For this review, take the finished solid that the model builds, in its own axes (mm). Coordinates: 2 decimals unless noted, no trailing zeros. Loops run counter-clockwise (first coordinate to the right, second up) from the corner with the lowest first, then second, coordinate; pieces in that order, holes last. Notation, with made-up numbers: (52, -30) - (87, -30) arc R16 ccw to (87, -23) - close; hole circle Ø4 at (62.5, 7.25). An arc over 180 degrees is marked (long way). Answer as a JSON object with one key per item and string values. Group by question number.
Item 1: We need section D-D (y = 5). State how many separate pieces and enclosed holes the cut face has, then the cut area to 3 significant figures.
Item 2: Clearance check with flat-ended pins moving along their axes: pin 1 (3.5 mm diameter, centred on y = 4.5, z = -31.5, fed in from -X); pin 2 (5 mm diameter, centred on y = 5, z = -90.52, fed in from -X); pin 3 (0.6 mm diameter, centred on x = -4.5, y = 3, fed in from +Z). State where each tip first meets the part, or that it passes through.
Item 3: We need section C-C (z = -28). Give the boundary of the cut face in (x, y), then the cut area to 3 significant figures.
Item 4: We need section B-B (z = -9). Give the boundary of the cut face in (x, y), then the cut area to 3 significant figures.
Item 5: To check wall thickness, follow line 1 (Y direction, x = 2.95, z = -90.52); line 2 (X direction, y = 3.5, z = -92); line 3 (X direction, y = 5.5, z = -7). State the ranges of each line that lie inside material, in increasing order.
Item 6: We need section A-A (z = -90.52). Give the boundary of the cut face in (x, y), then the cut area to 3 significant figures.
from build123d import *

# Parameters (mm, degrees)
SKETCH1_W                        = 5.5
SKETCH1_H                        = 11
MAIN_BASE_DEPTH                  = 96.52
SIDE_CUT_OUT_DEPTH               = 84.52
TOP_RUBBER_BAND_CUT_OUT_DEPTH    = 98.300361767
BOTTOM_RUBBER_BAND_CUT_OUT_DEPTH = 98.300361767
SKETCH6_W                        = 1.75
SKETCH6_H                        = 11
MOTOR_PULLEY_CUT_OUT_DEPTH       = 12
SKETCH7_W                        = 1.75
SKETCH7_H                        = 11
PULLEY_CUT_OUT_DEPTH             = 10
SKETCH11_R                       = 1.5
MOTOR_SHAFT_CUT_OUT_DEPTH        = 98.217143036
SKETCH17_W                       = 3.14
SKETCH17_H                       = 2.8
MOUNTING_POINTS_DEPTH            = 8.5
MOUNTING_POINTS_DRAFT            = -1.348
MOUNTING_POINTS_PROFILE_2_DEPTH  = 8.5
MOUNTING_POINTS_PROFILE_2_DRAFT  = -1.348
SKETCH13_W                       = 1
SKETCH13_H                       = 0.5
BOSS_EXTRUDE3_DEPTH              = 12
RAIL_CHAMFER_SIZE                = 0.5


with BuildPart() as part:
    # Sketch1 → main_base (new body)
    with BuildSketch(Plane.XY):
        with Locations((2.75, 5.5)):
            Rectangle(SKETCH1_W, SKETCH1_H)
    extrude(amount=-MAIN_BASE_DEPTH)

    # Sketch3 → side_cut_out (cut)
    with BuildSketch(Plane.XY):
        Polygon((5.5, 9), (3.5, 7), (3.5, 0), (5.5, 0), align=None)
    extrude(amount=-SIDE_CUT_OUT_DEPTH, mode=Mode.SUBTRACT)

    # Sketch4 → top_rubber_band_cut_out (cut, through all)
    with BuildSketch(Plane.XY):
        Polygon((0, 7.3), (0, 11), (2.7, 11), (2.7, 10), align=None)
    extrude(amount=-TOP_RUBBER_BAND_CUT_OUT_DEPTH, mode=Mode.SUBTRACT)

    # Sketch5 → bottom_rubber_band_cut_out (cut, through all)
    with BuildSketch(Plane.XY):
        Polygon((2, 0), (0, 2), (0, 0), align=None)
    extrude(amount=-BOTTOM_RUBBER_BAND_CUT_OUT_DEPTH, mode=Mode.SUBTRACT)

    # Sketch6 → motor_pulley_cut_out (cut)
    with BuildSketch(Plane(origin=(0, 0, -96.52), x_dir=(-1, 0, 0), z_dir=(0, 0, -1))):
        with Locations((-0.875, 5.5)):
            Rectangle(SKETCH6_W, SKETCH6_H)
    extrude(amount=-MOTOR_PULLEY_CUT_OUT_DEPTH, mode=Mode.SUBTRACT)

    # Sketch7 → pulley_cut_out (cut)
    with BuildSketch(Plane.XY):
        with Locations((0.875, 5.5)):
            Rectangle(SKETCH7_W, SKETCH7_H)
    extrude(amount=-PULLEY_CUT_OUT_DEPTH, mode=Mode.SUBTRACT)

    # Sketch10 → half_circle_cut_out (revolve, cut)
    with BuildSketch(Plane(origin=(0, 5, 0), x_dir=(1, 0, 0), z_dir=(0, 1, 0))):
        with BuildLine():
            Line((1.5, 5), (1.5, 3.75))
            ThreePointArc((1.5, 3.75), (2.383883476, 4.116116524), (2.75, 5))
            Line((2.75, 5), (1.5, 5))
        make_face()
    revolve(axis=Axis((2.75, 5, -5), (-1, 0, 0)), mode=Mode.SUBTRACT)

    # Sketch11 → motor_shaft_cut_out (cut, through all)
    with BuildSketch(Plane.ZY.offset(-1.75)):
        with Locations((-90.52, 5)):
            Circle(SKETCH11_R)
    extrude(amount=-MOTOR_SHAFT_CUT_OUT_DEPTH, mode=Mode.SUBTRACT)


with BuildPart() as mounting_points_tool:
    # Sketch17 → mounting_points (with draft: the straight prism first)
    with BuildSketch(Plane.XZ):
        with Locations((4.13, -0.15)):
            Rectangle(SKETCH17_W, SKETCH17_H)
    extrude(amount=-MOUNTING_POINTS_DEPTH)
    # mounting_points: the draft: its side faces are tilted about the plane it starts from
    mounting_points_sides = [mounting_points_tool.faces().sort_by_distance(p)[0] for p in [
        (4.13, 4.25, 1.25),
        (2.56, 4.25, -0.15),
        (4.13, 4.25, -1.55),
        (5.7, 4.25, -0.15),
    ]]
    draft(mounting_points_sides, Plane.XZ, MOUNTING_POINTS_DRAFT)


with BuildPart() as part_1:
    add(part.part)

    # mounting_points: cut by mounting_points_tool
    add(mounting_points_tool.part, mode=Mode.SUBTRACT)


with BuildPart() as mounting_points_profile_2_tool:
    # Sketch17 → mounting_points profile 2 (with draft: the straight prism first)
    with BuildSketch(Plane.XZ):
        with Locations((4.13, -96.37)):
            Rectangle(SKETCH17_W, SKETCH17_H)
    extrude(amount=-MOUNTING_POINTS_PROFILE_2_DEPTH)
    # mounting_points profile 2: the draft: its side faces are tilted about the plane it starts from
    mounting_points_profile_2_sides = [mounting_points_profile_2_tool.faces().sort_by_distance(p)[0] for p in [
        (4.13, 4.25, -97.77),
        (5.7, 4.25, -96.37),
        (4.13, 4.25, -94.97),
        (2.56, 4.25, -96.37),
    ]]
    draft(mounting_points_profile_2_sides, Plane.XZ, MOUNTING_POINTS_PROFILE_2_DRAFT)


with BuildPart() as part_2:
    add(part_1.part)

    # mounting_points profile 2: cut by mounting_points_profile_2_tool
    add(mounting_points_profile_2_tool.part, mode=Mode.SUBTRACT)

    # final_mirror: part across plane


with BuildPart() as part_3:
    add(part_2.part)
    add(part_2.part.mirror(Plane(origin=(0, 0, 0), x_dir=(0, 0, 1), z_dir=(1, 0, 0))))

    # Sketch13 → Boss-Extrude3 (add)
    with BuildSketch(Plane(origin=(0, 0, -96.52), x_dir=(-1, 0, 0), z_dir=(0, 0, -1))):
        Polygon((7.25, 11), (5.5, 11), (5.5, 10), (6.25, 10), (7.25, 10), align=None)
        with Locations((6.75, 9.75)):
            Rectangle(SKETCH13_W, SKETCH13_H)
    extrude(amount=-BOSS_EXTRUDE3_DEPTH)

    # rail_chamfer
    rail_chamfer_edges = [part_3.edges().sort_by_distance(p)[0] for p in [
        (-5.5, 11, -42.26),
        (-7.25, 11, -90.52),
        (5.5, 11, -48.26),
    ]]
    chamfer(rail_chamfer_edges, length=RAIL_CHAMFER_SIZE)


solid = part_3.part
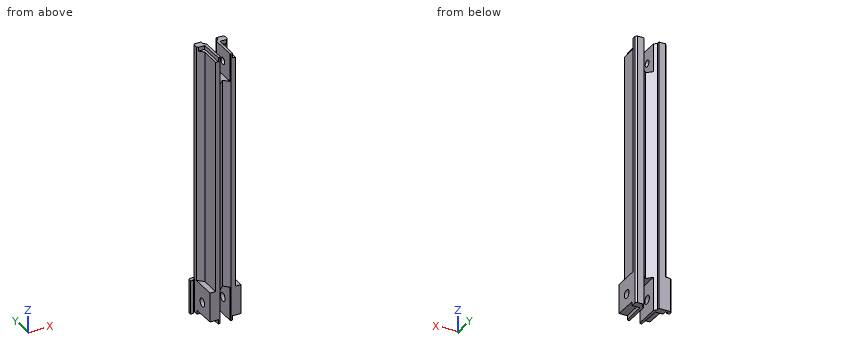
Check sheet entries:
{
 "1": {"separate pieces": "3", "enclosed holes": "0", "area": "610 mm2"},
 "2": {"pin 1": "stops at x = -3.5", "pin 2": "stops at x = -5.5", "pin 3": "stops at z = -84.52"},
 "3": {"outline": "(-5.5, 9) - (-3.5, 7) - (-3.5, 0) - (-2, 0) - (0, 2) - (2, 0) - (3.5, 0) - (3.5, 7) - (5.5, 9) - (5.5, 10.5) - (5, 11) - (2.7, 11) - (2.7, 10) - (0, 7.3) - (-2.7, 10) - (-2.7, 11) - (-5, 11) - (-5.5, 10.5) - close", "area": "72.1 mm2"},
 "4": {"outline": "(-5.5, 9) - (-3.5, 7) - (-3.5, 0) - (-2, 0) - (-1.75, 0.25) - (-1.75, 9.05) - (-2.7, 10) - (-2.7, 11) - (-5, 11) - (-5.5, 10.5) - close; (1.75, 0.25) - (2, 0) - (3.5, 0) - (3.5, 7) - (5.5, 9) - (5.5, 10.5) - (5, 11) - (2.7, 11) - (2.7, 10) - (1.75, 9.05) - close", "area": "47.4 mm2"},
 "5": {"line 1": "y = 0 to 3.5, 6.5 to 11", "line 2": "x = -5.5 to -1.75, 1.75 to 5.5", "line 3": "x = -3.5 to -1.75, 1.75 to 3.5"},
 "6": {"outline": "(-7.25, 9.5) - (-6.25, 9.5) - (-6.25, 10) - (-5.5, 10) - (-5.5, 6.5) - (-1.75, 6.5) - (-1.75, 9.05) - (-2.7, 10) - (-2.7, 11) - (-6.75, 11) - (-7.25, 10.5) - close; (-5.5, 0) - (-2, 0) - (-1.75, 0.25) - (-1.75, 3.5) - (-5.5, 3.5) - close; (1.75, 0.25) - (2, 0) - (5.5, 0) - (5.5, 3.5) - (1.75, 3.5) - close; (1.75, 6.5) - (5.5, 6.5) - (5.5, 10.5) - (5, 11) - (2.7, 11) - (2.7, 10) - (1.75, 9.05) - close", "area": "59.1 mm2"}
}
